The figure shows three views and two pictorial views of one solid part (mm, origin at its lowest corner). Answer the questions. Give positions to 0.01 mm unless a question says otherwise; leave off trailing zeros. Order: outer loops, then holes, each group sorted by start corner. A loop starts at its lowest first (then second) coordinate and runs counter-clockwise, first axis right, second up. Notation, with made-up numbers: (87, 42.25) -> (116, 42.25) arc R9 cw to (116, 58.25) -> close; hole circle Ø7 at (59, 53.5). An arc over 180 degrees is marked (long way). One line per item, written item: value. Start each with the question number.
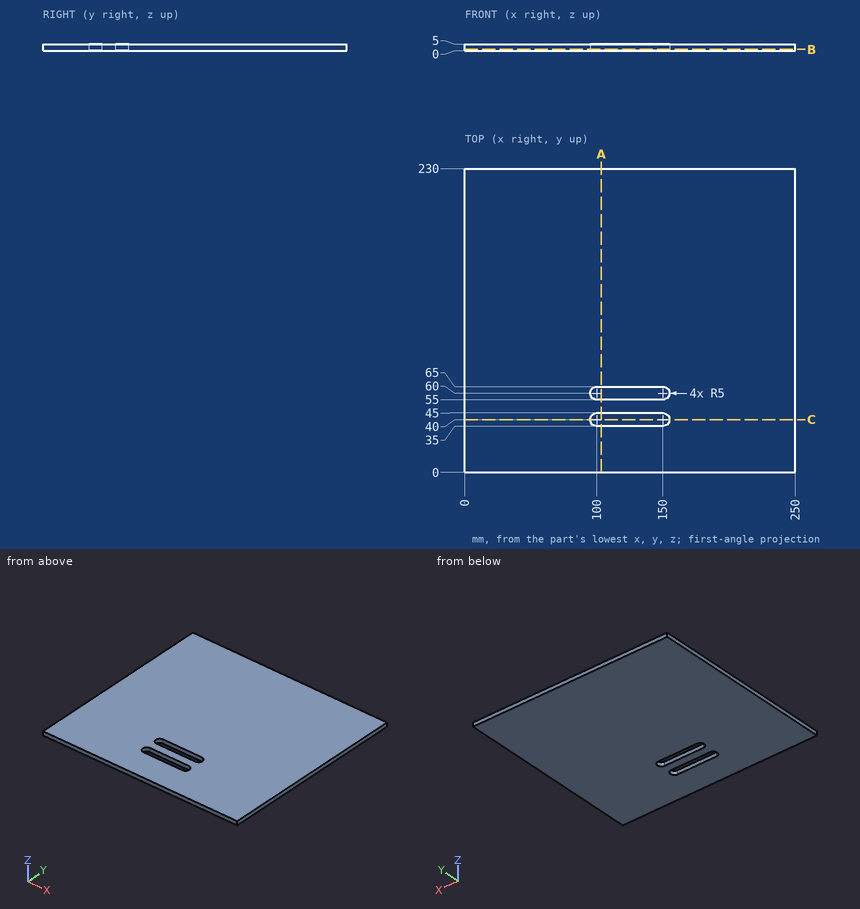
Item 1: A flat-ended cylindrical pin translates along its axis: pin 1 (1 mm diameter, centred on y = 158.5, z = 3.5, fed in from -X). Find the tip coordinate at first contact, or state that the pin passes through.
Item 2: Find section C-C on y = 40. Write down the section's boundary in (x, z).
Item 3: Find section A-A on x = 103.5. Write down the section's boundary in (y, z), then the cut area to 3 significant figures.
Item 4: Find the intervals of material crossed by line 1 (Y direction, x = 109, z = 2.95); line 2 (Y direction, x = 98.5, z = 0.9), in increasing order. Write a range as from..to.
Item 5: Find section B-B on z = 0.95. Write down the section's boundary in (x, y), then the cut area to 3 significant figures.
Checks:
1. pin 1: x = 0
2. outline: (0, 0) -> (95, 0) -> (95, 5) -> (0, 5) -> close; (155, 0) -> (250, 0) -> (250, 5) -> (155, 5) -> close
3. outline: (0, 0) -> (35, 0) -> (35, 5) -> (0, 5) -> close; (45, 0) -> (55, 0) -> (55, 5) -> (45, 5) -> close; (65, 0) -> (230, 0) -> (230, 5) -> (65, 5) -> close
3. area: 1,050 mm2
4. line 1: 0..35, 45..55, 65..230
4. line 2: 0..35.23, 44.77..55.23, 64.77..230
5. outline: (0, 0) -> (250, 0) -> (250, 230) -> (0, 230) -> close; hole (100, 35) -> (150, 35) arc R5 ccw to (150, 45) -> (100, 45) arc R5 ccw to start; hole (100, 55) -> (150, 55) arc R5 ccw to (150, 65) -> (100, 65) arc R5 ccw to start
5. area: 56,300 mm2
